Drawing for the job (mm, zero at the part's lowest x, y, z). Give positions to 0.01 mm unless a question says otherwise; leave off trailing zeros. Order: outer loops, then holes, each group sorted by start corner. A loop starts at its lowest first (then second) coordinate and runs counter-clockwise, first axis right, second up. Notation, with made-up numbers: (-25, 3.25) - (34, 3.25) arc R21 ccw to (34, 10.25) - close; hole circle Ø10 at (-17.5, 49). An arc over 180 degrees is marked (long way). Use a Markdown table: item, result.
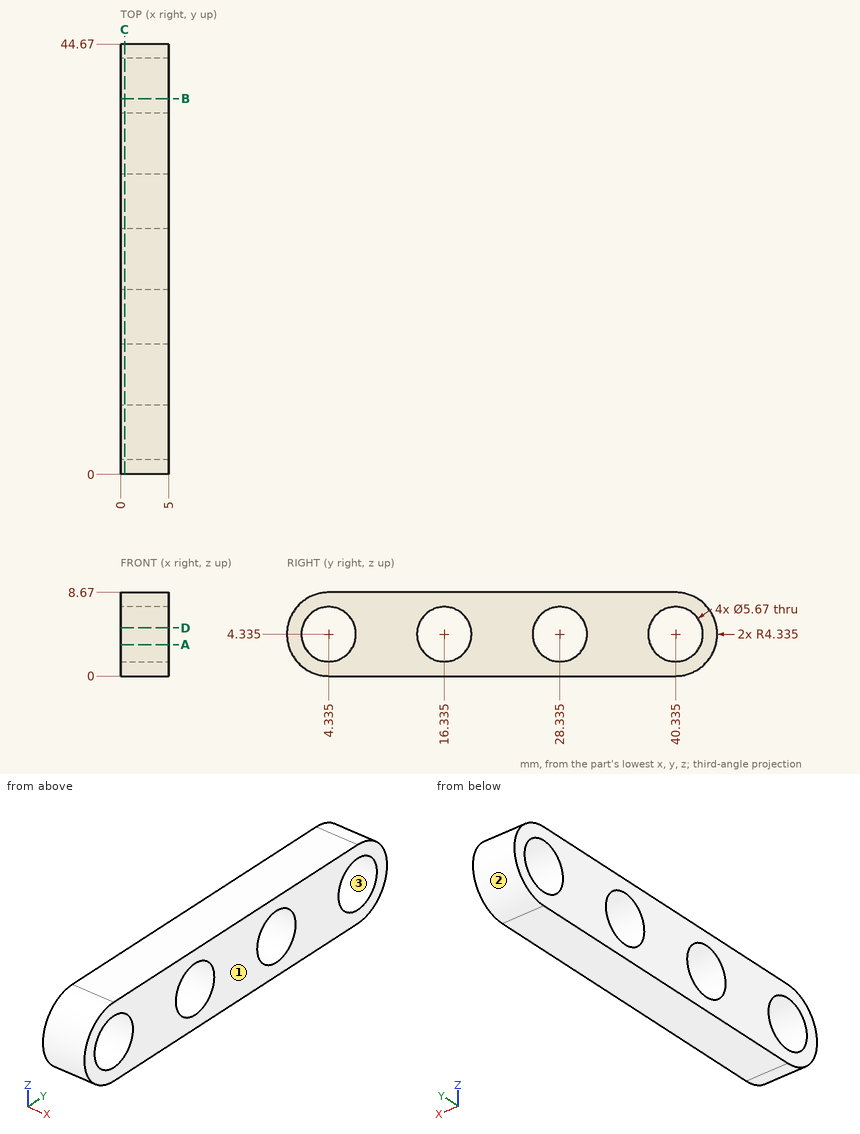
1) Pin check, flat tips, straight feed: P1, Ø2, axis at x = 3, z = 2.5, coming from the +Y side; P2, Ø1.5, axis at x = 4, z = 6.5, coming from the -Y side. Stop position of each tip, or through.
Computed:
| item | result |
|---|---|
| P1 | stops at y = 44.59 |
| P2 | stops at y = 0.24 |
2) Slice it at C-C (x = 0.4). Write the cut outline in (y, z) (3 decimals).
Computed:
| item | result |
|---|---|
| outline | (4.335, 0) - (40.335, 0) arc R4.335 ccw to (40.335, 8.67) - (4.335, 8.67) arc R4.335 ccw to start; hole circle Ø5.67 at (4.335, 4.335); hole circle Ø5.67 at (16.335, 4.335); hole circle Ø5.67 at (28.335, 4.335); hole circle Ø5.67 at (40.335, 4.335) |
3) Wall check: line 1 (Y direction, x = 3.85, z = 4.25); line 2 (Y direction, x = 4.65, z = 3); line 3 (Z direction, x = 4.2, y = 5). Give the ranges that are in metal, low to high. Write a range as from..to.
Computed:
| item | result |
|---|---|
| line 1 | y = 0..1.5, 7.17..13.5, 19.17..25.5, 31.17..37.5, 43.17..44.67 |
| line 2 | y = 0.21..1.83, 6.84..13.83, 18.84..25.83, 30.84..37.83, 42.84..44.46 |
| line 3 | z = 0..1.58, 7.09..8.67 |
4) Slice it at B-B (y = 39). Write the cut outline in (x, z), and give its area (3 significant figures).
Computed:
| item | result |
|---|---|
| outline | (0, 0) - (5, 0) - (5, 1.83) - (0, 1.83) - close; (0, 6.84) - (5, 6.84) - (5, 8.67) - (0, 8.67) - close |
| area | 18.3 mm² |
5) Slice it at A-A (z = 3.25). Write the cut outline in (x, y), and give its area (3 significant figures).
Computed:
| item | result |
|---|---|
| outline | (0, 0.14) - (5, 0.14) - (5, 1.72) - (0, 1.72) - close; (0, 6.95) - (5, 6.95) - (5, 13.72) - (0, 13.72) - close; (0, 18.95) - (5, 18.95) - (5, 25.72) - (0, 25.72) - close; (0, 30.95) - (5, 30.95) - (5, 37.72) - (0, 37.72) - close; (0, 42.95) - (5, 42.95) - (5, 44.53) - (0, 44.53) - close |
| area | 117 mm² |
6) Two-plate mould, pull along Z, no slides. Class the marked faces 1, 2 and 3: +Z half, -Z half, draft (parallel to the pull), parting line (faces both ways), or undercut.
Computed:
| item | result |
|---|---|
| face 1 | draft |
| face 2 | parting line |
| face 3 | undercut |
7) Slice it at D-D (z = 5). Write the cut outline in (x, y).
Computed:
| item | result |
|---|---|
| outline | (0, 0.05) - (5, 0.05) - (5, 1.58) - (0, 1.58) - close; (0, 7.09) - (5, 7.09) - (5, 13.58) - (0, 13.58) - close; (0, 19.09) - (5, 19.09) - (5, 25.58) - (0, 25.58) - close; (0, 31.09) - (5, 31.09) - (5, 37.58) - (0, 37.58) - close; (0, 43.09) - (5, 43.09) - (5, 44.62) - (0, 44.62) - close |
